The model under review builds one solid part; all positions refer to its coordinate system, in mm. A direction names the side the tool comes from. Round coordinates to 2 decimals unless told otherwise and drop trailing zeros. Order: outer loops, then holes, each group sorted by start corner. A loop starts at its lowest first (then second) coordinate and runs counter-clockwise, first axis right, second up. Notation, with made-up numbers: M -27,76 L 10,76 A17 ccw 10,97 Z; hole C 0.5,-39.75 d9. An arc over 180 degrees is marked long. One line per item, written item: value. Start each with the question number.
from build123d import *

# Parameters (mm, degrees)
F1_DEPTH  = 19.05
F3_DEPTH  = 50.8
F6_DEPTH  = 1.27
F7_DEPTH  = 1.27
F9_DEPTH  = 4.064
F11_DEPTH = 3.81
F12_W     = 30.4800014411
F12_H     = 35.6379195737
F13_DEPTH = 3.81
F14_R     = 0.1905
F15_DEPTH = 1.016
F17_DEPTH = 50.8
F18_R     = 0.4693884444
F18_R_2   = 0.3677883594
F19_DEPTH = 38.0999
F20_DEPTH = 42.8752


with BuildPart() as f1:
    # F0 (on Right) → F1 (new body, symmetric)
    with BuildSketch(Plane.YZ):
        Polygon((-4.300991216, 39.0530479294), (-38.9073263628, -3.5559992527), (4.3505917698, -3.5559992527), align=None)
        Polygon((-6.2876227312, 30.9665426612), (0, 0), (-31.4381159842, 0), align=None, mode=Mode.SUBTRACT)
    extrude(amount=F1_DEPTH, both=True)

    # F2 (on face) → F3 (cut)
    with BuildSketch(Plane.YZ.offset(19.05)):
        Polygon((-6.3284697347, 36.5567151771), (-3.7941216332, 36.5567151771), (-4.300991216, 39.0530479294), align=None)
    extrude(amount=-F3_DEPTH, mode=Mode.SUBTRACT)

    # F5 (on face) → F6 (join)
    with BuildSketch(Plane(origin=(-19.05, 0, 0), x_dir=(0, -1, 0), z_dir=(-1, 0, 0))):
        Polygon((5.7698168155, 28.4163484679), (2.1412553343, 28.4163484679), (2.1412553343, 25.6189145148), (5.2018099345, 25.6189145148), align=None)
        Polygon((8.3588465857, 28.4163484679), (5.7698168155, 28.4163484679), (5.2018099345, 25.6189145148), (10.6308743201, 25.6189145148), align=None)
        Polygon((12.9399355427, 28.4163484679), (8.3588465857, 28.4163484679), (10.6308743201, 25.6189145148), (13.2188182324, 25.6189145148), (13.2188182324, 28.0729741801), align=None)
    extrude(amount=F6_DEPTH)

    # F4 (on face) → F7 (join)
    with BuildSketch(Plane.YZ.offset(19.05)):
        Polygon((-8.4918548826, 28.2525820137), (-13.0729438396, 28.2525820137), (-13.0729438396, 25.6189145148), (-10.6308743201, 25.6189145148), align=None)
        Polygon((-2.2463577334, 28.2525820137), (-5.7365647443, 28.2525820137), (-5.2018099345, 25.6189145148), (-2.2463577334, 25.6189145148), align=None)
        Polygon((-5.7365647443, 28.2525820137), (-8.4918548826, 28.2525820137), (-10.6308743201, 25.6189145148), (-5.2018099345, 25.6189145148), align=None)
    extrude(amount=F7_DEPTH)

    # F8 (on face) → F9 (cut)
    with BuildSketch(Plane(origin=(0, -21.7030111813, 17.6268123393), x_dir=(1, 0, 0), z_dir=(0, -0.7762344906, 0.6304443002))):
        Polygon((-15.2399991697, 13.4574822013), (-15.2399991697, -23.4791905796), (15.2399991697, -23.4791905796), (15.2399991697, 13.688865676), (15.2399991697, 13.8253802434), (15.2399991697, 20.5768346786), (-15.2399991697, 20.5768346786), (-15.2399991697, 13.8998411689), align=None)
    extrude(amount=-F9_DEPTH, mode=Mode.SUBTRACT)

    # F10 (on face) → F11 (cut)
    with BuildSketch(Plane(origin=(0, 3.4848880888, 0.7075914739), x_dir=(-1, 0, 0), z_dir=(0, 0.9800024806, 0.1989852707))):
        Polygon((15.2400027211, 32.7706485987), (-15.2400027211, 32.7706485987), (-15.2400027211, -0.5405944909), (15.2400027211, -0.5405944909), (15.2400027211, 28.2741702614), align=None)
    extrude(amount=-F11_DEPTH, mode=Mode.SUBTRACT)

    # F12 (on face) → F13 (cut)
    with BuildSketch(Plane(origin=(0, 0, -3.5559992527), x_dir=(1, 0, 0), z_dir=(0, 0, -1))):
        with Locations((0, 17.2783672965)):
            Rectangle(F12_W, F12_H)
    extrude(amount=-F13_DEPTH, mode=Mode.SUBTRACT)

    # F14 (on face) → F15 (join)
    with BuildSketch(Plane(origin=(0, -21.7030111813, 17.6268123393), x_dir=(1, 0, 0), z_dir=(0, -0.7762344906, 0.6304443002))):
        with Locations((-17.1998851001, 22.4818350938)):
            Circle(F14_R)
        with Locations((17.1449995848, 22.4818350938)):
            Circle(F14_R)
    extrude(amount=F15_DEPTH)

    # F16 (on face) → F17 (cut)
    with BuildSketch(Plane.YZ.offset(19.05)):
        Polygon((-38.9073263628, -3.5559992527), (-36.8760041893, -3.5559992527), (-36.8760041893, -1.0549340007), align=None)
    extrude(amount=-F17_DEPTH, mode=Mode.SUBTRACT)

    # F18 (on face) → F19 (join)
    with BuildSketch(Plane(origin=(-19.05, 0, 0), x_dir=(0, -1, 0), z_dir=(-1, 0, 0))):
        with Locations((8.2998776285, 35.7320597078)):
            Circle(F18_R)
        with Locations((8.2998776285, 35.7320597078)):
            Circle(F18_R_2, mode=Mode.SUBTRACT)
    extrude(amount=-F19_DEPTH)

    # F18 (on face) → F20 (cut)
    with BuildSketch(Plane(origin=(-19.05, 0, 0), x_dir=(0, -1, 0), z_dir=(-1, 0, 0))):
        with Locations((8.2998776285, 35.7320597078)):
            Circle(F18_R_2)
    extrude(amount=-F20_DEPTH, mode=Mode.SUBTRACT)


solid = f1.part
Item 1: Wall thickness on L1, parallel to X at y = -3.5, z = 31; L2, parallel to Y at x = 15.5, z = 28; L3, parallel to Y at x = 6, z = -1: over which ranges is each line inside the solid? List them lowest first.
Item 2: Clearance check with flat-ended pins moving along their axes: P1, Ø1, axis at x = 0.5, z = 1.5, coming from the +Y side; P2, Ø3, axis at x = 1, z = -1.5, coming from the +Y side; P3, Ø3, axis at x = 10, y = -10, coming from the +Z side; P4, Ø1.9, axis at y = -15.5, z = -2, coming from the -X side. State where each tip first meets the part, or that it passes through.
Item 3: The part is to be moulded in two halves that separate along X. For faces 5 (the flat face through (-20, -8, 25.619)), 6 (the flat face through (-20.32, -8, 27)), 7 (the flat face through (0, 0.541, -2)), say which applies: pulls with the +X half, pulls with the -X half, needs draft (parallel to the pull), parting line crosses it, or undercut.
Item 4: Consider section B-B, the plane x = 11.5. Give the boundary of the cut face in (y, z).
Item 5: Consider section A-A, the plane y = -16.5. Give the boundary of the cut face in (x, z), then the cut area to 3 significant figures.
Item 6: Machinability: for faces 1 (the flat face through (20, -13.073, 27)), 2 (the flat face through (19.05, -7, 27)), 3 (the flat face through (-20, -2.141, 27)), 4 (the flat face through (-20, -8, 28.416)), which of the approach directions +Z, -Z, +X, -X, +Y, -Y give a long, thin tool a straight path to every point of the face, cutting with its end or side? Answer none if there is none.
Item 7: Consider section C-C, the plane z = 10.5. Give the boundary of the cut face in (x, y).
Computed:
1. L1: x = -19.05 to -15.24, 15.24 to 19.05
1. L2: y = -13.28 to -8.7, -5.69 to -2.06
1. L3: y = -36.83 to -36.01, 0.54 to 3.83
2. P1: passes through
2. P2: stops at y = 4.24
2. P3: stops at z = 36.16
2. P4: stops at x = -19.05
3. face 5: needs draft
3. face 6: pulls with the -X half
3. face 7: undercut
4. outline: M -36.88,-3.56 L -35.1,-3.56 L -35.1,-1.74 L -36.51,-0.6 L -36.88,-1.05 Z; C -8.3,35.73 d0.94; M -8.73,33.6 L -6.76,32 L -6.77,32.06 L -3.04,32.82 L -3.79,36.56 L -6.33,36.56 Z; M 0.54,-3.56 L 4.35,-3.56 L 3.59,0.18 L 0.54,-0.44 Z; hole C -8.3,35.73 d0.74
5. outline: M -19.05,-3.56 L -15.24,-3.56 L -15.24,0 L -19.05,0 Z; M -19.05,18.39 L -15.24,18.39 L -15.24,24.03 L -19.05,24.03 Z; M 15.24,-3.56 L 19.05,-3.56 L 19.05,0 L 15.24,0 Z; M 15.24,18.39 L 19.05,18.39 L 19.05,24.03 L 15.24,24.03 Z
5. area: 70.1 mm^2
6. face 1: +Z, -Z, +X, -Y
6. face 2: none
6. face 3: +Z, -Z, -X, +Y
6. face 4: +Z, -X, +Y, -Y
7. outline: M -19.05,-27.49 L -15.24,-27.49 L -15.24,-22.91 L -19.05,-22.91 Z; M -19.05,-2.13 L -15.24,-2.13 L -15.24,1.5 L -19.05,1.5 Z; M 15.24,-27.49 L 19.05,-27.49 L 19.05,-22.91 L 15.24,-22.91 Z; M 15.24,-2.13 L 19.05,-2.13 L 19.05,1.5 L 15.24,1.5 Z
